Work out the finished part from the listing and answer in its coordinate system (mm). A direction names the side the tool comes from. Coordinates: 2 decimals unless noted, no trailing zeros. Loops run counter-clockwise (first coordinate to the right, second up) from the corner with the lowest first, then second, coordinate; pieces in that order, holes last. Notation, with made-up numbers: (84, 88.25) - (138, 88.25) arc R30 cw to (138, 110.25) - close; hole circle Ø3 at (76, -7.75). An arc over 180 degrees is marked (long way). Write each question's results on one line, items separated by ' | '. Start each with the question number.
Item 1: Section B-B, the plane z = -25.5 is taken. Write down the section's boundary in (x, y), plus the area to 3 significant figures.
Item 2: For a pull along Y with two mould halves and no side action, classify faces 4 (the face through (40.286, 49.096, 10.027)), 5 (the face through (38.116, 61.405, -15.027)), 6 (the face through (27.84, -0.722, 0.47)), 7 (the face through (23, 31, 33.6)) as +Y half, -Y half, draft (parallel to the pull), parting line (faces both ways), or undercut.
Item 3: A tool of negligible diameter and unlimited length cuts with its end or side. For faces 1 (the face through (42.11, 34.38, 0.45)), 2 (the face through (39, 55, 6.25)), 3 (the face through (38.116, 61.405, 14.973)), from which of +Z, -Z, +X, -X, +Y, -Y can it reach the whole face along a straight path? Write none if from no direction.
Item 4: Section A-A, the plane x = 33.5 is taken. Write down the section's boundary in (y, z), plus the area to 3 significant figures.
Item 5: Section D-D, the plane z = 5 is taken. Write down the section's boundary in (x, y).
Item 6: Consider probe 1 along Z at (x, y) = (30, 19); probe 2 along Y at (x, z) = (15, 11); probe 3 along Y at (x, z) = (10.5, -8). Determine where each line is inside the solid, lowest interval first. Write a range as [from, to].
Item 7: Section C-C, the plane y = 13.5 is taken. Write down the section's boundary in (x, z), plus the area to 3 significant figures.
Item 8: Each of these flat-tipped pins is pushed along its axis until it touches: pin 1 Ø5 at (y, z) = (35, -13) entering from -X; pin 2 Ø8 at (x, z) = (36.5, -16) entering from -Y; pin 3 Ø4 at (x, z) = (37, 2.5) entering from -Y. Where does it stop, or does it pass through?
Autodesk Fusion 360 part; units mm, degrees
sketch "Sketch1" plane through (0, 0, 0) normal (0, 0, 1) x (1, 0, 0)
  line L0 (7.1104, -4.3777) -> (49.1586, 3.0365)
  line L1 (49.1586, 3.0365) -> (38.1927, 65.227)
  line L2 (38.1927, 65.227) -> (7.1104, 65.227)
  line L3 (7.1104, 65.227) -> (7.1104, -4.3777)
  line L4 (7.1104, 63.727) -> (12.1104, 63.727)
  line L5 (12.1104, 63.727) -> (12.1104, -1.973)
  line L6 (12.1104, -1.973) -> (7.1104, -1.973)
  line L7 (12.1104, 62.727) -> (37.1104, 62.727)
  line L8 (37.1104, 62.727) -> (47.2499, 5.2231)
  line L9 (47.2499, 5.2231) -> (12.1104, -0.973)
  dimension "d5" = 80
  dimension "d6" = 1.5
  dimension "d8" = 5
  dimension "d9" = 65.7
  dimension "d11" = 1.5
  dimension "d12" = 1
  dimension "d13" = 1
  dimension "d40" = 1.5
  dimension "d41" = 30
extrude "Extrude4" add sketch "Sketch1" against normal blind 32.1 contours L3 L4 L5 L6 | L5 L7 L8 L9 makes body 1
extrude "Extrude3" add sketch "Sketch1" along normal blind 32.1 separate body contours L3 L4 L5 L6 | L5 L7 L8 L9 makes body 2
extrude "Extrude1" add sketch "Sketch1" along normal blind 33.6 separate body makes body 3
extrude "Extrude2" add 1 faces at (21.1265, 21.2953, 0) along direction (0, 0, -1) blind 33.6 on bodies 3 bodies 3
combine "Combine1" operation add target body 1 tool bodies 2
combine "Combine2" operation cut target body 3 tool bodies 1
sketch "Sketch2" plane through (0, 0, -33.6) normal (0, 0, -1) x (-1, 0, 0)
  line L0 (-7.1104, -4.3777) -> (-7.1104, 65.227)
  line L1 (-7.1104, 65.227) -> (-38.1927, 65.227)
  line L2 (-38.1927, 65.227) -> (-49.1586, 3.0365)
  line L3 (-49.1586, 3.0365) -> (-7.1104, -4.3777)
  line L4 (-7.1104, 8.6223) -> (-15.1104, 8.6223)
  line L5 (-17.1104, 6.6223) -> (-17.1104, 5.6223)
  line L6 (-15.1104, 3.6223) -> (-7.1104, 3.6223)
  arc A0 (-15.1104, 8.6223) -> (-17.1104, 6.6223) centre (-15.1104, 6.6223) ccw
  arc A1 (-17.1104, 5.6223) -> (-15.1104, 3.6223) centre (-15.1104, 5.6223) ccw
  line L7 (-7.1104, 65.227) -> (-7.1104, -4.3777)
  dimension "d23" = 2
  dimension "d24" = 2
  dimension "d26" = 8
  dimension "d27" = 10
  dimension "d28" = 5
extrude "Extrude5" cut sketch "Sketch2" against normal blind 1.5 contours L0 L4 L5 L6 A0 A1 L7 bodies 3
sketch "Sketch3" plane through (48.1956, 8.4982, 0) normal (0.9848, 0.1736, 0) x (0, 0, -1)
  line L0 (33.6, 57.604) -> (-33.6, 57.604)
  line L1 (-33.6, 57.604) -> (-33.6, -5.546)
  line L2 (-33.6, -5.546) -> (33.6, -5.546)
  line L3 (33.6, -5.546) -> (33.6, 57.604)
  line L4 (1.25, 42.604) -> (1.25, 52.604)
  arc A0 (1.25, 52.604) -> (-1.25, 52.604) centre (0, 52.604) ccw
  line L5 (-1.25, 52.604) -> (-1.25, 42.604)
  arc A1 (-1.25, 42.604) -> (1.25, 42.604) centre (0, 42.604) ccw
  line L6 (0, 42.604) -> (0, 52.604) construction
  line L7 (0, 57.604) -> (0, 47.604) construction
  arc A2 (-13.75, 52.604) -> (-16.25, 52.604) centre (-15, 52.604) ccw
  arc A3 (-16.25, 42.604) -> (-13.75, 42.604) centre (-15, 42.604) ccw
  line L8 (-13.75, 42.604) -> (-13.75, 52.604)
  line L9 (-16.25, 52.604) -> (-16.25, 42.604)
  arc A4 (-8.75, 52.604) -> (-11.25, 52.604) centre (-10, 52.604) ccw
  arc A5 (-11.25, 42.604) -> (-8.75, 42.604) centre (-10, 42.604) ccw
  line L10 (-8.75, 42.604) -> (-8.75, 52.604)
  line L11 (-11.25, 52.604) -> (-11.25, 42.604)
  arc A6 (-3.75, 52.604) -> (-6.25, 52.604) centre (-5, 52.604) ccw
  arc A7 (-6.25, 42.604) -> (-3.75, 42.604) centre (-5, 42.604) ccw
  line L12 (-3.75, 42.604) -> (-3.75, 52.604)
  line L13 (-6.25, 52.604) -> (-6.25, 42.604)
  arc A8 (6.25, 52.604) -> (3.75, 52.604) centre (5, 52.604) ccw
  arc A9 (3.75, 42.604) -> (6.25, 42.604) centre (5, 42.604) ccw
  line L14 (6.25, 42.604) -> (6.25, 52.604)
  line L15 (3.75, 52.604) -> (3.75, 42.604)
  arc A10 (11.25, 52.604) -> (8.75, 52.604) centre (10, 52.604) ccw
  arc A11 (8.75, 42.604) -> (11.25, 42.604) centre (10, 42.604) ccw
  line L16 (11.25, 42.604) -> (11.25, 52.604)
  line L17 (8.75, 52.604) -> (8.75, 42.604)
  arc A12 (16.25, 52.604) -> (13.75, 52.604) centre (15, 52.604) ccw
  arc A13 (13.75, 42.604) -> (16.25, 42.604) centre (15, 42.604) ccw
  line L18 (16.25, 42.604) -> (16.25, 52.604)
  line L19 (13.75, 52.604) -> (13.75, 42.604)
  point P0 (0, 47.604)
  dimension "d31" = 2.5
  dimension "d32" = 10
  dimension "d33" = 10
  dimension "d36" = 5
  dimension "d37" = 0
extrude "Extrude6" cut sketch "Sketch3" against normal blind 1.5 contours L4 A0 L5 A1 | A2 A3 L8 L9 | A4 A5 L10 L11 | A6 A7 L12 L13 | A8 A9 L14 L15 | A10 A11 L16 L17 | A12 A13 L18 L19 bodies 3
equation "wall_thickness = 1.5 mm"
equation "d6 = wall_thickness"
equation "d9 = 64.2 mm + wall_thickness"
equation "d11 = wall_thickness"
equation "d14 = 32.1 mm + wall_thickness"
equation "d16 = 32.1 mm + wall_thickness"
equation "d40 = wall_thickness"
Answer key:
1) outline: (7.11, -4.38) - (49.16, 3.04) - (38.19, 65.23) - (7.11, 65.23) - (7.11, 63.73) - (12.11, 63.73) - (12.11, 62.73) - (37.11, 62.73) - (47.25, 5.22) - (12.11, -0.97) - (12.11, -1.97) - (7.11, -1.97) - close | area: 263 mm^2
2) face 4: +Y half | face 5: undercut | face 6: -Y half | face 7: draft
3) face 1: -X | face 2: +X, -X | face 3: +X
4) outline: (0.28, -33.6) - (65.23, -33.6) - (65.23, 33.6) - (0.28, 33.6) - close; hole (2.8, -32.1) - (62.73, -32.1) - (62.73, 32.1) - (2.8, 32.1) - close | area: 517 mm^2
5) outline: (7.11, -4.38) - (49.16, 3.04) - (41.01, 49.22) - (39.54, 48.96) - (47.25, 5.22) - (12.11, -0.97) - (12.11, -1.97) - (7.11, -1.97) - close; (7.11, 63.73) - (12.11, 63.73) - (12.11, 62.73) - (37.11, 62.73) - (37.37, 61.27) - (38.84, 61.53) - (38.19, 65.23) - (7.11, 65.23) - close
6) probe 1: z = [-33.6, -32.1], [32.1, 33.6] | probe 2: y = [-2.99, -0.46], [62.73, 65.23] | probe 3: y = [-3.78, -1.97], [63.73, 65.23]
7) outline: (7.11, -33.6) - (47.31, -33.6) - (47.31, 33.6) - (7.11, 33.6) - (7.11, 32.1) - (45.79, 32.1) - (45.79, -32.1) - (7.11, -32.1) - close | area: 218 mm^2
8) pin 1: stops at x = 41.56 | pin 2: stops at y = 0.1 | pin 3: stops at y = 0.54
